Read the model definition and answer for the solid it produces. Units are mm, in the model's axes. A direction names the side the tool comes from. Round coordinates to 2 decimals unless told otherwise and drop trailing zeros. Loops run counter-clockwise (first coordinate to the right, second up) from the corner with the lowest first, then second, coordinate; pieces in that order, holes last. Notation, with made-up numbers: (69.25, -0.5) - (111.25, -0.5) arc R18 ccw to (111.25, 25.5) - close; hole circle Ø5 at (83, -18). An arc over 180 degrees is marked (long way). Use CSV: the item, a comma, the result in double quotes. Start each with the question number.
1. Find section D-D (z = 11.5). Give the vertices of the cut face in (x, y), and give its area (3 significant figures).
2. Determine the mould class of faces 6 (the flat face through (0, 0, 6)), 7 (the cylindrical face through (-11.107, 1.479, 26.789)), 8 (the flat face through (0, 4, -3.556)) for opening direction Z: +Z half, -Z half, draft (parallel to the pull), parting line (faces both ways), or undercut.
3. Find section B-B (z = 0). Give the vertices of the cut face in (x, y).
4. Consider line 1 along Z through (x, y) = (2.5, 9.75); line 2 along X through (y, z) = (6.5, -4.35) (3 decimals); line 3 along Y through (x, z) = (0, 4.65) (3 decimals). Determine where each line is inside the solid, lowest interval first.
5. Find section C-C (y = 1.25). Give the vertices of the cut face in (x, z), and give its area (3 significant figures).
6. Given pin 1 Ø2 at (x, y) = (0.5, 5) entering from -Z; pin 2 Ø17.5 at (x, z) = (9, -11.5) entering from +Y; pin 3 Ø1.5 at (y, z) = (5.5, 4.5) entering from -X, each flat-ended and moving along its own axis, determine where each tip first touches the part or whether it passes through.
7. A tool of negligible diameter and unlimited length cuts with its end or side. For faces 1 (the flat face through (4.5, 5, -5)), 2 (the flat face through (-4.5, 5, 5)), 3 (the flat face through (0, 4, -6.556)), 4 (the flat face through (0, 4, 3.556)), 5 (the flat face through (0, 4, 6.556)), from which of +Z, -Z, +X, -X, +Y, -Y can it reach the whole face along a straight path? Write none if from no direction.
8. Find section A-A (x = 0). Give the vertices of the cut face in (y, z) (3 decimals), and give its area (4 significant figures).
from build123d import *

# Parameters (mm, degrees)
SKETCH1_R               = 29
SKETCH1_R_2             = 3.5
BOSS_EXTRUDE1_DEPTH     = 3
SKETCH2_W               = 9
SKETCH2_H               = 3
BOSS_EXTRUDE2_DEPTH     = 7
CUT_EXTRUDE1_DEPTH      = 43.213741838
CUT_EXTRUDE1_DEPTH_BACK = 43.213741838
SKETCH4_R               = 2.125
CUT_EXTRUDE4_START      = -6.555610355
CUT_EXTRUDE4_DEPTH      = 13.11122071


# Read off the part's stored shape, not the designer's step: Cut-Extrude4
with BuildPart() as part:
    # Sketch1 → Boss-Extrude1 (new body)
    with BuildSketch(Plane(origin=(0, 0, 0), x_dir=(1, 0, 0), z_dir=(0, 1, 0))):
        with Locations(Location((0, 0, 0), (0, 0, 270))):
            Circle(SKETCH1_R)
        with Locations(Location((0, 0, 0), (0, 0, 270))):
            Circle(SKETCH1_R_2, mode=Mode.SUBTRACT)
    extrude(amount=BOSS_EXTRUDE1_DEPTH)

    # Sketch2 → Boss-Extrude2 (add)
    with BuildSketch(Plane(origin=(0, 3, 0), x_dir=(1, 0, 0), z_dir=(0, 1, 0))):
        with Locations((0, 5.055610355)):
            Rectangle(SKETCH2_W, SKETCH2_H)
        with Locations((0, -5.055610355)):
            Rectangle(SKETCH2_W, SKETCH2_H)
    extrude(amount=BOSS_EXTRUDE2_DEPTH)

    # Sketch4 → Cut-Extrude1 (cut, two sides: drawn at the far end of the back side and taken through both)
    with BuildSketch(Plane.XY.offset(-CUT_EXTRUDE1_DEPTH_BACK)):
        with Locations((0, 6.5)):
            Circle(SKETCH4_R)
    extrude(amount=CUT_EXTRUDE1_DEPTH + CUT_EXTRUDE1_DEPTH_BACK, mode=Mode.SUBTRACT)

    # Cut-Extrude4 outline → Cut-Extrude4 (cut)
    with BuildSketch(Plane.XY.offset(CUT_EXTRUDE4_START)):
        with BuildLine():
            Line((4.5, 10), (1.5, 10))
            ThreePointArc((1.5, 10), (3.621320344, 9.121320344), (4.5, 7))
            Line((4.5, 7), (4.5, 10))
        make_face()
        with BuildLine():
            ThreePointArc((-4.5, 7), (-3.621320344, 9.121320344), (-1.5, 10))
            Line((-1.5, 10), (-4.5, 10))
            Line((-4.5, 10), (-4.5, 7))
        make_face()
    extrude(amount=CUT_EXTRUDE4_DEPTH, mode=Mode.SUBTRACT)


solid = part.part
Filled sheet:
1,outline,"(-26.62, 0) - (26.62, 0) - (26.62, 3) - (-26.62, 3) - close"
1,area,"160 mm²"
2,face 6,"draft"
2,face 7,"parting line"
2,face 8,"undercut"
3,outline,"(-29, 0) - (-3.5, 0) - (-3.5, 3) - (-29, 3) - close; (3.5, 0) - (29, 0) - (29, 3) - (3.5, 3) - close"
4,line 1,"z = -6.56 to -3.56, 3.56 to 6.56"
4,line 2,"x = -4.5 to -2.125, 2.125 to 4.5"
4,line 3,"y = 0 to 4.375, 8.625 to 10"
5,outline,"circle Ø58 at (0, 0); hole circle Ø7 at (0, 0)"
5,area,"2,600 mm²"
6,pin 1,"stops at z = -6.56"
6,pin 2,"stops at y = 9.99"
6,pin 3,"stops at x = -4.5"
7,face 1,"+Z, -Z, +X, +Y"
7,face 2,"+Z, -Z, -X, +Y"
7,face 3,"-Z, +X, -X, +Y"
7,face 4,"+X, -X, +Y"
7,face 5,"+Z, +X, -X, +Y"
8,outline,"(0, -29) - (3, -29) - (3, -6.556) - (4.375, -6.556) - (4.375, -3.556) - (3, -3.556) - (3, -3.5) - (0, -3.5) - close; (0, 3.5) - (3, 3.5) - (3, 3.556) - (4.375, 3.556) - (4.375, 6.556) - (3, 6.556) - (3, 29) - (0, 29) - close; (8.625, -6.556) - (10, -6.556) - (10, -3.556) - (8.625, -3.556) - close; (8.625, 3.556) - (10, 3.556) - (10, 6.556) - (8.625, 6.556) - close"
8,area,"169.5 mm²"
